The figure shows three views and two pictorial views of one solid part (mm, origin at its lowest corner). Answer the questions. Give positions to 0.01 mm unless a question says otherwise; leave off trailing zeros. Order: outer loops, then holes, each group sorted by start corner. A loop starts at its lowest first (then second) coordinate and runs counter-clockwise, first axis right, second up. Notation, with made-up numbers: (-6.5, -5) - (39.5, -5) arc R19 cw to (39.5, 2) - close; hole circle Ø11 at (-8.75, 32.25). An arc over 180 degrees is marked (long way). Answer as CSV lines item,"result". Start each with the question number.
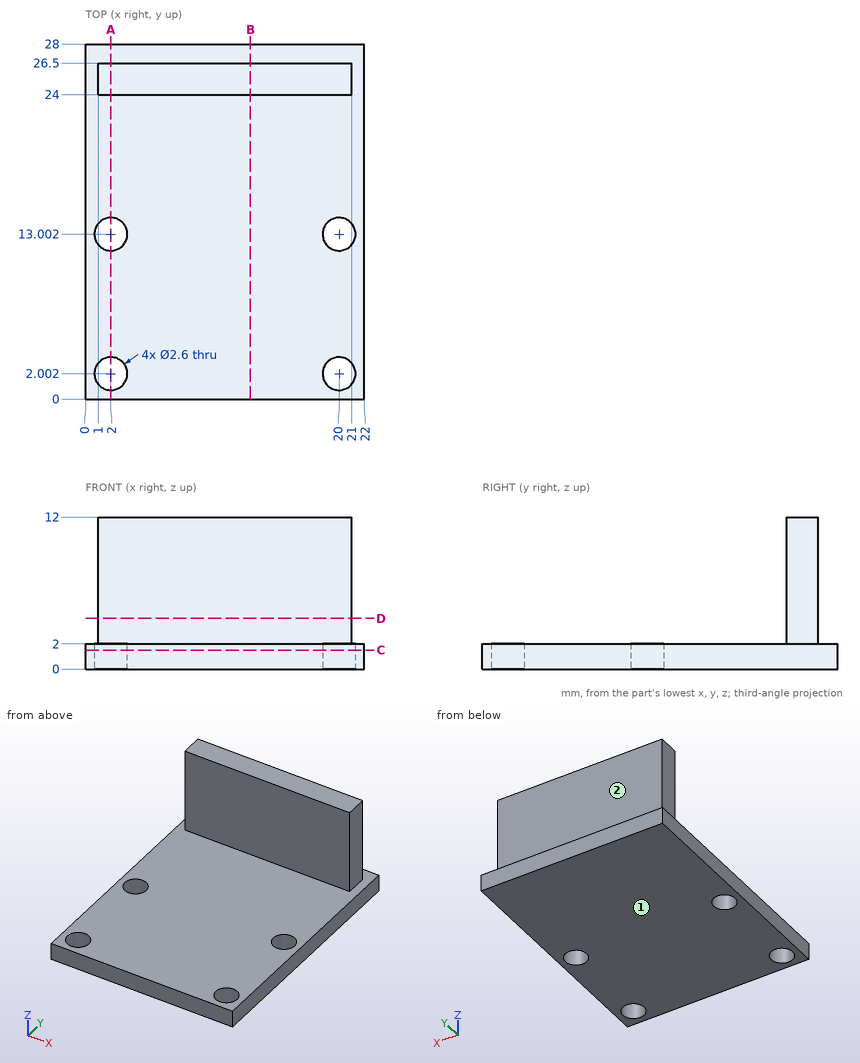
(1) Determine the mould class of the marked faces 1 and 2 for opening direction Z: released by +Z, released by -Z, zero draft, split by the parting line, or undercut.
(2) Section A-A, the plane x = 2 is taken. Write down the section's boundary in (y, z), and give its area (3 significant figures).
(3) Section C-C, the plane z = 1.5 is taken. Write down the section's boundary in (x, y), and give its area (3 significant figures).
(4) Section D-D, the plane z = 4 is taken. Write down the section's boundary in (x, y), and give its area (3 significant figures).
(5) Straight lines are drawn through the part: line 1 (Y direction, x = 2, z = 0.45); line 2 (X direction, y = 26, z = 6.5); line 3 (Y direction, x = 18, z = 10.5). For each, find the intervals that lie inside material, in ascending order. Write a range as [from, to].
(6) Section B-B, the plane x = 13 is taken. Write down the section's boundary in (y, z).
(7) Flat-ended cylindrical pins translate along their axes: pin 1 Ø2 at (x, y) = (3, 3) entering from -Z; pin 2 Ø3 at (x, z) = (15.5, 4.5) entering from -Y; pin 3 Ø3 at (y, z) = (25, 7.5) entering from -X; pin 4 Ø2 at (y, z) = (25.5, 9.5) entering from +X. Find the tip coordinate at first contact, or state that the pin passes through.
Checks:
1,face 1,"released by -Z"
1,face 2,"zero draft"
2,outline,"(0, 0) - (0.7, 0) - (0.7, 2) - (0, 2) - close; (3.3, 0) - (11.7, 0) - (11.7, 2) - (3.3, 2) - close; (14.3, 0) - (28, 0) - (28, 2) - (26.5, 2) - (26.5, 12) - (24, 12) - (24, 2) - (14.3, 2) - close"
2,area,"70.6 mm²"
3,outline,"(0, 0) - (22, 0) - (22, 28) - (0, 28) - close; hole circle Ø2.6 at (2, 2); hole circle Ø2.6 at (2, 13); hole circle Ø2.6 at (20, 2); hole circle Ø2.6 at (20, 13)"
3,area,"595 mm²"
4,outline,"(1, 24) - (21, 24) - (21, 26.5) - (1, 26.5) - close"
4,area,"50.0 mm²"
5,line 1,"y = [0, 0.7], [3.3, 11.7], [14.3, 28]"
5,line 2,"x = [1, 21]"
5,line 3,"y = [24, 26.5]"
6,outline,"(0, 0) - (28, 0) - (28, 2) - (26.5, 2) - (26.5, 12) - (24, 12) - (24, 2) - (0, 2) - close"
7,pin 1,"stops at z = 0"
7,pin 2,"stops at y = 24"
7,pin 3,"stops at x = 1"
7,pin 4,"stops at x = 21"
